Study the drawing (mm; zero at the part's minimum x, y, z) and answer. A direction names the side the tool comes from. Give positions to 0.01 mm unless a question says otherwise; leave off trailing zeros. Write each loop counter-clockwise with the first axis right and the second up, starting at its lowest first coordinate (ties: lowest second). Pieces come first, ordered by that corner, then holes.
1) Given pin 1 Ø1.9 at (x, z) = (19.5, 4.5) entering from +Y, flat-ended and moving along its own axis, determine where the tip first touches the part or whether it passes through.
2) Find section B-B (y = 12). Determine the outline of the cut face in (x, z) (3 decimals), plus the area to 3 significant figures.
3) Find section A-A (y = 4.5). Determine the outline of the cut face in (x, z) (3 decimals), plus the area to 3 significant figures.
4) Find section C-C (x = 37). Determine the outline of the cut face in (y, z).
5) A tool of negligible diameter and unlimited length cuts with its end or side. For the marked faces 1 and 2, from which of +Z, -Z, +X, -X, +Y, -Y can it reach the whole face along a straight path? Write none if from no direction.
6) Straight lines are drawn through the part: probe 1 along X at (y, z) = (19, 3); probe 2 along Y at (x, z) = (6.5, 0.5); probe 3 along X at (y, z) = (12, 2.75). For each, find the intervals that lie inside material, in ascending order.
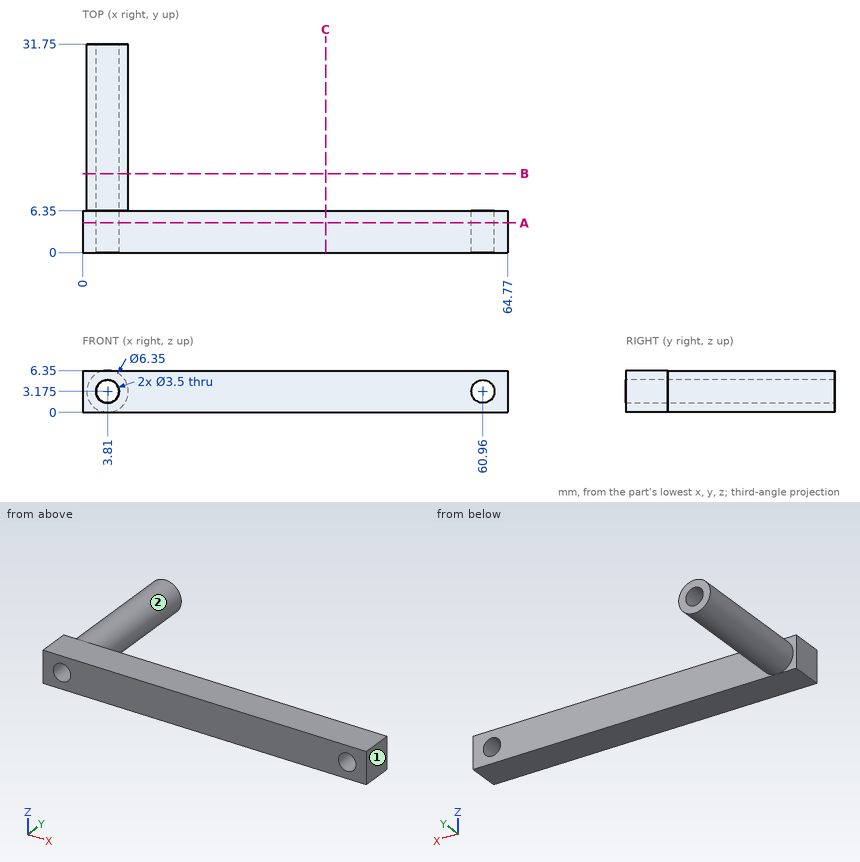
Results:
1. pin 1: stops at y = 6.35
2. outline: circle Ø6.35 at (3.81, 3.175); hole circle Ø3.5 at (3.81, 3.175)
2. area: 22.0 mm2
3. outline: (0, 0) - (64.77, 0) - (64.77, 6.35) - (0, 6.35) - close; hole circle Ø3.5 at (3.81, 3.175); hole circle Ø3.5 at (60.96, 3.175)
3. area: 392 mm2
4. outline: (0, 0) - (6.35, 0) - (6.35, 6.35) - (0, 6.35) - close
5. face 1: +Z, -Z, +X, +Y, -Y
5. face 2: +Y
6. probe 1: x = 0.64 to 2.07, 5.55 to 6.98
6. probe 2: y = 0 to 6.35
6. probe 3: x = 0.66 to 2.11, 5.51 to 6.96
